Could you check a few things on this model? Use its own coordinates, in mm. A direction names the side the tool comes from. Round coordinates to 2 decimals unless told otherwise and drop trailing zeros. Loops run counter-clockwise (first coordinate to the right, second up) from the corner with the lowest first, then second, coordinate; pieces in that order, holes last. Notation, with made-up numbers: (35, 43.25) -> (66, 43.25) arc R30 ccw to (66, 68.25) -> close; hole circle Ø7 at (40.25, 44). An arc over 180 degrees is marked (long way). Put each result on its own line as item: value. Start each with the question number.
1. Imagine slicing it at D-D, the plane x = 33.5. Please give me the cut outline in (y, z).
2. I'm going to push a flat-ended pin straight in: P1, Ø0.6, axis at x = 7.5, z = 1, coming from the -Y side. Where does the tip first touch, or does it pass through?
3. I need wall thicknesses on line 1 (X direction, y = 1.25, z = 0.4); line 2 (Y direction, x = 21, z = 0.6); line 3 (Y direction, x = 22, z = 0.5). Which ranges of each line are inside material? Lowest first, please. Write a range as [from, to].
4. If we mould it in two halves opening along Y, with no side actions, what happens to faces 1 (the flat face through (9.574, 13.938, 0.986)), 2 (the flat face through (13.771, 8.235, 0.986)), 3 (the cylindrical face through (24.98, 15.98, 0.99)), 4 (the flat face through (31, 1, 1))? For each: pulls with the +Y half, pulls with the -Y half, needs draft (parallel to the pull), parting line crosses it, or undercut.
5. Which directions (+Z, -Z, +X, -X, +Y, -Y) give clear straight access to the entire face, cutting with the end or side of a thin tool? Please do faces 5 (the flat face through (10, 3, 1)), 6 (the cylindrical face through (35.844, 4.311, 0.986)).
6. Imagine slicing it at B-B, the plane z = 0.85. Please give me the cut outline in (x, y), and give its area (3 significant figures).
7. Imagine slicing it at A-A, the plane x = 22. Please give me the cut outline in (y, z).
8. Imagine slicing it at C-C, the plane y = 20. Please give me the cut outline in (x, z).
```python
from build123d import *

# Parameters (mm, degrees)
SKETCH1_R           = 1.75
BOSS_EXTRUDE1_DEPTH = 2


with BuildPart() as part:
    # Sketch1 → Boss-Extrude1 (new body)
    with BuildSketch(Plane.XY):
        with BuildLine():
            Line((0, 0), (0, 3.535533906))
            ThreePointArc((0, 3.535533906), (0.152240935, 4.300900771), (0.585786438, 4.949747468))
            Line((0.585786438, 4.949747468), (18.818019485, 23.181980515))
            ThreePointArc((18.818019485, 23.181980515), (25.089650716, 23.271705741), (25.358752948, 17.005208082))
            ThreePointArc((25.358752948, 17.005208082), (24.978951169, 15.964033329), (25.417677093, 14.946283938))
            Line((25.417677093, 14.946283938), (35.414213562, 4.949747468))
            ThreePointArc((35.414213562, 4.949747468), (35.847759065, 4.300900771), (36, 3.535533906))
            Line((36, 3.535533906), (36, 0))
            Line((36, 0), (31, 0))
            Line((31, 0), (31, 2))
            Line((31, 2), (26, 2))
            Line((26, 2), (26, 3.73959236))
            ThreePointArc((26, 3.73959236), (25.866789182, 4.409288367), (25.487436867, 4.977029227))
            Line((25.487436867, 4.977029227), (19.060660172, 11.403805922))
            ThreePointArc((19.060660172, 11.403805922), (18, 11.843145751), (16.939339828, 11.403805922))
            Line((16.939339828, 11.403805922), (10.512563133, 4.977029227))
            ThreePointArc((10.512563133, 4.977029227), (10.133210818, 4.409288367), (10, 3.73959236))
            Line((10, 3.73959236), (10, 2))
            Line((10, 2), (5, 2))
            Line((5, 2), (5, 0))
            Line((5, 0), (0, 0))
        make_face()
        with Locations((22, 20)):
            Circle(SKETCH1_R, mode=Mode.SUBTRACT)
    extrude(amount=BOSS_EXTRUDE1_DEPTH)


solid = part.part
```
Entries:
1. outline: (0, 0) -> (6.86, 0) -> (6.86, 2) -> (0, 2) -> close
2. P1: y = 2
3. line 1: [0, 5], [31, 36]
3. line 2: [9.46, 18.56], [21.44, 24.39]
3. line 3: [8.46, 18.25], [21.75, 24.5]
4. face 1: pulls with the +Y half
4. face 2: pulls with the -Y half
4. face 3: undercut
4. face 4: needs draft
5. face 5: +Z, -Z, -Y
5. face 6: +Z, -Z, +X, +Y
6. outline: (0, 0) -> (5, 0) -> (5, 2) -> (10, 2) -> (10, 3.74) arc R1.75 cw to (10.51, 4.98) -> (16.94, 11.4) arc R1.5 cw to (19.06, 11.4) -> (25.49, 4.98) arc R1.75 cw to (26, 3.74) -> (26, 2) -> (31, 2) -> (31, 0) -> (36, 0) -> (36, 3.54) arc R2 ccw to (35.41, 4.95) -> (25.42, 14.95) arc R1.5 cw to (25.36, 17.01) arc R4.5 ccw to (18.82, 23.18) -> (0.59, 4.95) arc R2 ccw to (0, 3.54) -> close; hole circle Ø3.5 at (22, 20)
6. area: 359 mm^2
7. outline: (8.46, 0) -> (18.25, 0) -> (18.25, 2) -> (8.46, 2) -> close; (21.75, 0) -> (24.5, 0) -> (24.5, 2) -> (21.75, 2) -> close
8. outline: (15.64, 0) -> (20.25, 0) -> (20.25, 2) -> (15.64, 2) -> close; (23.75, 0) -> (26.5, 0) -> (26.5, 2) -> (23.75, 2) -> close
